Could you check a few things on this model? Use its own coordinates, in mm. Face numbers are marked on the shaded views. A direction names the side the tool comes from. Round coordinates to 2 decimals unless told otherwise and drop trailing zeros. Loops run counter-clockwise (first coordinate to the right, second up) from the corner with the lowest first, then second, coordinate; pieces in that order, holes last. Notation, with made-up numbers: (74.5, 36) -> (122.5, 36) arc R19 ccw to (122.5, 54) -> close; hole circle Ø8 at (19, 61). An arc over 180 degrees is marked (long way). Write each question's results on one line, items separated by ' | '.
from build123d import *

# Parameters (mm, degrees)
SKETCH1_R           = 12.7
SKETCH1_R_2         = 6.35
BOSS_EXTRUDE1_DEPTH = 5.08
SKETCH2_R           = 9.525
SKETCH2_R_2         = 6.35
BOSS_EXTRUDE2_DEPTH = 27.6225
SKETCH3_OUTSIDE_W   = 37.116
SKETCH3_OUTSIDE_H   = 37.116
SKETCH3_OUTSIDE_R   = 7.4676
CUT_EXTRUDE1_DEPTH  = 0.9906
SKETCH5_R           = 28.575
BOSS_EXTRUDE4_DEPTH = 6.587499906
BOSS_EXTRUDE5_DEPTH = 15.875
SKETCH12_W          = 57.15
SKETCH12_H          = 9.779
CUT_EXTRUDE2_DEPTH  = 16.1125
BOSS_EXTRUDE6_DEPTH = 15.875


with BuildPart() as part:
    # Sketch1 → Boss-Extrude1 (new body)
    with BuildSketch(Plane(origin=(0, 0, 0), x_dir=(1, 0, 0), z_dir=(0, 1, 0))):
        Circle(SKETCH1_R)
        Circle(SKETCH1_R_2, mode=Mode.SUBTRACT)
    extrude(amount=BOSS_EXTRUDE1_DEPTH)

    # Sketch2 → Boss-Extrude2 (add)
    with BuildSketch(Plane(origin=(0, 5.08, 0), x_dir=(1, 0, 0), z_dir=(0, 1, 0))):
        Circle(SKETCH2_R)
        Circle(SKETCH2_R_2, mode=Mode.SUBTRACT)
    extrude(amount=BOSS_EXTRUDE2_DEPTH)

    # Sketch3 outside → Cut-Extrude1 (cut)
    with BuildSketch(Plane(origin=(0, 16.1925, 0), x_dir=(-1, 0, 0), z_dir=(0, 1, 0))):
        Rectangle(SKETCH3_OUTSIDE_W, SKETCH3_OUTSIDE_H)
        Circle(SKETCH3_OUTSIDE_R, mode=Mode.SUBTRACT)
    extrude(amount=CUT_EXTRUDE1_DEPTH, mode=Mode.SUBTRACT)

    # Sketch5 → Boss-Extrude4 (add)
    with BuildSketch(Plane.XZ):
        Circle(SKETCH5_R)
    extrude(amount=BOSS_EXTRUDE4_DEPTH)

    # Sketch8 → Boss-Extrude5 (add)
    with BuildSketch(Plane.XZ.offset(6.587499906)):
        with BuildLine():
            Line((23.759524406, -15.875), (-23.759524406, -15.875))
            ThreePointArc((-23.759524406, -15.875), (0, -28.575), (23.759524406, -15.875))
        make_face()
        with BuildLine():
            ThreePointArc((23.759524406, 15.875), (0, 28.575), (-23.759524406, 15.875))
            Line((-23.759524406, 15.875), (23.759524406, 15.875))
        make_face()
    extrude(amount=BOSS_EXTRUDE5_DEPTH)

    # Sketch12 → Cut-Extrude2 (cut)
    with BuildSketch(Plane(origin=(0, 0, 0), x_dir=(1, 0, 0), z_dir=(0, 1, 0))):
        with Locations((0, 23.6855)):
            Rectangle(SKETCH12_W, SKETCH12_H)
        with Locations((0, -23.6855)):
            Rectangle(SKETCH12_W, SKETCH12_H)
    extrude(amount=-CUT_EXTRUDE2_DEPTH, mode=Mode.SUBTRACT)

    # Sketch13 → Boss-Extrude6 (add)
    with BuildSketch(Plane.XZ.offset(6.587499906)):
        with BuildLine():
            Line((23.759524406, 15.875), (-23.759524406, 15.875))
            ThreePointArc((-23.759524406, 15.875), (-28.575, 0), (-23.759524406, -15.875))
            Line((-23.759524406, -15.875), (23.759524406, -15.875))
            ThreePointArc((23.759524406, -15.875), (28.575, 0), (23.759524406, 15.875))
        make_face()
    extrude(amount=BOSS_EXTRUDE6_DEPTH)


solid = part.part
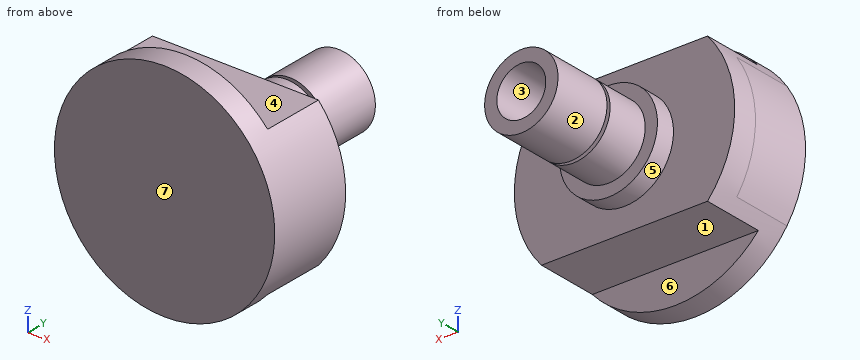
1) I need wall thicknesses on line 1 (Z direction, x = 0, y = 20) (3 decimals); line 2 (Y direction, x = 12, z = 23). Which ranges of each line are inside material? Lowest first, please.
Model answer:
line 1: z = -9.525 to -6.35, 6.35 to 9.525 | line 2: y = -22.46 to -16.11
2) I want a section at B-B, the plane y = 9. Write out the boundary of the cut face in (x, z) (3 decimals).
Model answer:
outline: circle Ø19.05 at (0, 0); hole circle Ø12.7 at (0, 0)
3) I'm going to push flat-ended pins straight in: pin 1 (10 mm diameter, centred on x = 13, y = 16, fed in from +Z); pin 2 (3 mm diameter, centred on x = -9.5, z = -24, fed in from +Y); pin 3 (6 mm diameter, centred on x = -2.5, y = 7, fed in from -Z). Where does each tip first touch, or does it pass through?
Model answer:
pin 1: stops at z = 5.17 | pin 2: stops at y = -16.11 | pin 3: stops at z = -12.7
4) I want a section at C-C, the plane x = -16.5. Write out the boundary of the cut face in (y, z).
Model answer:
outline: (-22.46, -23.33) -> (-16.11, -23.33) -> (-16.11, -18.8) -> (0, -18.8) -> (0, 18.8) -> (-16.11, 18.8) -> (-16.11, 23.33) -> (-22.46, 23.33) -> close
5) I want a section at D-D, the plane z = 21.5. Write out the boundary of the cut face in (x, y).
Model answer:
outline: (-18.82, -22.46) -> (18.82, -22.46) -> (18.82, -16.11) -> (-18.82, -16.11) -> close
6) If we mould it in two halves opening along Z, with no side actions, what happens to the marked faces 1, 2, 3 and 4? For each: released by +Z, released by -Z, zero draft, split by the parting line, or undercut.
Model answer:
face 1: released by -Z | face 2: split by the parting line | face 3: undercut | face 4: released by +Z
7) For the marked faces 5, 6 and 7, which set-ups out of +Z, -Z, +X, -X, +Y, -Y let a thin tool reach every point of the face, with its end or its side?
Model answer:
face 5: +Y | face 6: -Z, +X, -X, +Y | face 7: +Z, -Z, +X, -X, -Y
